from build123d import *

# Parameters (mm, degrees)
SKETCH1_W           = 3.5
SKETCH1_H           = 3.8
BOSS_EXTRUDE1_DEPTH = 3.6
SKETCH2_R           = 1.75
SKETCH2_R_2         = 1.35
BOSS_EXTRUDE2_DEPTH = 3
SKETCH3_W           = 0.5
SKETCH3_H           = 0.5
BOSS_EXTRUDE3_DEPTH = 3


with BuildPart() as part:
    # Sketch1 → Boss-Extrude1 (new body)
    with BuildSketch(Plane(origin=(0, 0, 0), x_dir=(1, 0, 0), z_dir=(0, 1, 0))):
        Rectangle(SKETCH1_W, SKETCH1_H)
    extrude(amount=BOSS_EXTRUDE1_DEPTH)

    # Sketch2 → Boss-Extrude2 (add)
    with BuildSketch(Plane(origin=(1.75, 0, 0), x_dir=(0, 0, -1), z_dir=(1, 0, 0))):
        with Locations(Location((0, 1.8, 0), (0, 0, 180))):
            Circle(SKETCH2_R)
        with Locations((0, 1.8)):
            Circle(SKETCH2_R_2, mode=Mode.SUBTRACT)
    extrude(amount=BOSS_EXTRUDE2_DEPTH)

    # Sketch3 → Boss-Extrude3 (add)
    with BuildSketch(Plane.XZ):
        with Locations((-1.27, 1.27)):
            Rectangle(SKETCH3_W, SKETCH3_H)
        with Locations((-1.27, -1.27)):
            Rectangle(SKETCH3_W, SKETCH3_H)
        with Locations((1.27, 1.27)):
            Rectangle(SKETCH3_W, SKETCH3_H)
        with Locations((1.27, -1.27)):
            Rectangle(SKETCH3_W, SKETCH3_H)
    extrude(amount=BOSS_EXTRUDE3_DEPTH)


solid = part.part
Here's how the part is built. I have some questions about the finished solid (model axes, mm). A direction names the side the tool comes from. Round coordinates to 2 decimals unless told otherwise and drop trailing zeros. Write each loop counter-clockwise with the first axis right and the second up, starting at its lowest first coordinate (ties: lowest second). Pieces come first, ordered by that corner, then holes. Notation, with made-up numbers: (-11.5, -37.75) -> (7.5, -37.75) arc R25 cw to (7.5, -14.75) -> close; hole circle Ø6 at (54, 52.25). An arc over 180 degrees is marked (long way). One line per item, written item: value.
1) Suppose I cut it at D-D on x = 2.75. List the corners of the cut face in (y, z) for me.
Filled sheet:
outline: circle Ø3.5 at (1.8, 0); hole circle Ø2.7 at (1.8, 0)
2) We'd pull the mould along Z, two halves only. Please class faces 1 (the face through (0, 0, 0)), 2 (the face through (1.75, 2, 0)), 3 (the face through (4.75, 3, 1)), 4 (the face through (0, 2, 1.9)): released by +Z, released by -Z, zero draft, split by the parting line, or undercut.
Filled sheet:
face 1: undercut
face 2: undercut
face 3: zero draft
face 4: released by +Z
3) Suppose I cut it at C-C on z = 0. List the corners of the cut face in (x, y) for me.
Filled sheet:
outline: (-1.75, 0) -> (1.75, 0) -> (1.75, 0.05) -> (4.75, 0.05) -> (4.75, 0.45) -> (1.75, 0.45) -> (1.75, 3.15) -> (4.75, 3.15) -> (4.75, 3.55) -> (1.75, 3.55) -> (1.75, 3.6) -> (-1.75, 3.6) -> close
4) Suppose I cut it at B-B on y = 1.8. List the corners of the cut face in (x, z) for me, plus the area to 3 significant figures.
Filled sheet:
outline: (-1.75, -1.9) -> (1.75, -1.9) -> (1.75, -1.75) -> (4.75, -1.75) -> (4.75, -1.35) -> (1.75, -1.35) -> (1.75, 1.35) -> (4.75, 1.35) -> (4.75, 1.75) -> (1.75, 1.75) -> (1.75, 1.9) -> (-1.75, 1.9) -> close
area: 15.7 mm2
5) For faces 5 (the face through (-1.75, 2, 0)), 6 (the face through (3.229, 3.139, 0.176)), which set-ups out of +Z, -Z, +X, -X, +Y, -Y let a thin tool reach every point of the face, with its end or its side?
Filled sheet:
face 5: +Z, -Z, -X, +Y, -Y
face 6: +X
6) I'm going to push flat-ended pins straight in: pin 1 Ø1 at (x, z) = (3, -1) entering from +Y; pin 2 Ø0.6 at (y, z) = (-1.5, 1) entering from -X; pin 3 Ø1.5 at (x, y) = (3.5, 1) entering from -Z. Where does each tip first touch, or does it pass through?
Filled sheet:
pin 1: stops at y = 3.48
pin 2: stops at x = -1.52
pin 3: stops at z = -1.75
7) Suppose I cut it at A-A on y = -1.75. List the corners of the cut face in (x, z) for me, plus the area to 3 significant figures.
Filled sheet:
outline: (-1.52, -1.52) -> (-1.02, -1.52) -> (-1.02, -1.02) -> (-1.52, -1.02) -> close; (-1.52, 1.02) -> (-1.02, 1.02) -> (-1.02, 1.52) -> (-1.52, 1.52) -> close; (1.02, -1.52) -> (1.52, -1.52) -> (1.52, -1.02) -> (1.02, -1.02) -> close; (1.02, 1.02) -> (1.52, 1.02) -> (1.52, 1.52) -> (1.02, 1.52) -> close
area: 1.00 mm2
8) If I drill on line 1 (X direction, y = -1, z = -1.15); line 2 (Y direction, x = 2.75, z = 0); line 3 (X direction, y = 1.5, z = -0.5), over which ranges is the centre line in solid material (lowest first)? Write a range as [from, to].
Filled sheet:
line 1: x = [-1.52, -1.02], [1.02, 1.52]
line 2: y = [0.05, 0.45], [3.15, 3.55]
line 3: x = [-1.75, 1.75]
